Verification items for the finished model (mm, model axes). Face numbers are marked on the shaded views. A direction names the side the tool comes from. Round coordinates to 2 decimals unless told otherwise and drop trailing zeros. Write each loop counter-clockwise with the first axis right and the second up, starting at its lowest first coordinate (ties: lowest second). Pieces come first, ordered by that corner, then holes. Notation, with made-up numbers: M 41.5,4.5 L 83.5,4.5 A20 cw 83.5,39.5 Z; hole C -8,-14 d3. An arc over 180 degrees is marked long. One line per item, written item: value. Start each with the question number.
from build123d import *

# Parameters (mm, degrees)
F0_W     = 19.2
F0_H     = 100
F1_DEPTH = 19.2
F2_W     = 15.4
F2_H     = 15.4
F3_DEPTH = 18
F4_SIZE  = 0.5


# Not quite as in the source:
# - a pattern or mirror of a feature is missing from the dataset's text; its kind, count and spacing are read off the source's solid


with BuildPart() as f1:
    # F0 (on Top) → F1 (new body)
    with BuildSketch(Plane.XY):
        Rectangle(F0_W, F0_H)
    extrude(amount=F1_DEPTH)

    # F2 (on face) → F3 (cut)
    with BuildSketch(Plane.YZ.offset(9.6)):
        with Locations((-40.4, 9.6)):
            Rectangle(F2_W, F2_H)
    f3 = extrude(amount=-F3_DEPTH, mode=Mode.SUBTRACT)

    # F3_copies: F3 across plane
    add(f3.mirror(Plane.ZX), mode=Mode.SUBTRACT)

    # F4
    f4_edges = [f1.edges().sort_by_distance(p)[0] for p in [
        (-9.6, 50, 9.6),
        (-9.6, -50, 9.6),
        (-9.6, 0, 0),
        (-9.6, 0, 19.2),
        (0, -50, 19.2),
        (9.6, 0, 19.2),
        (0, 50, 19.2),
        (9.6, -50, 9.6),
        (0, -50, 0),
        (9.6, 0, 0),
        (0, 50, 0),
        (9.6, 50, 9.6),
    ]]
    chamfer(f4_edges, length=F4_SIZE)


solid = f1.part
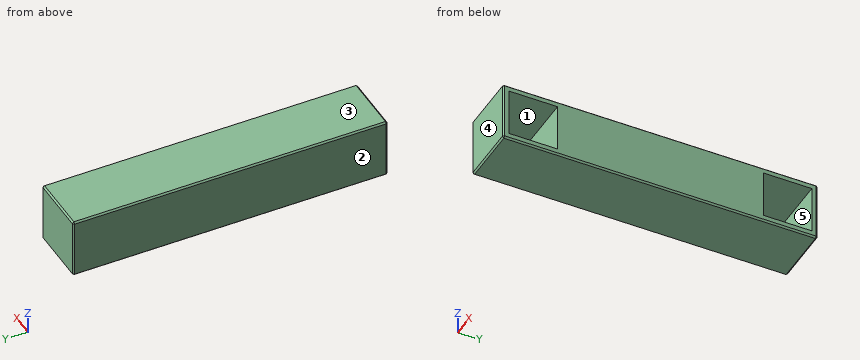
1) Cross-section at C-C (z = 13). Record the boundary of the cut face in (x, y).
2) Thickness scan on line 1 (Y direction, x = 7, z = 6); line 2 (Z direction, x = 3.75, y = 40). Record the ranges inside material, lowest first.
3) Cross-section at A-A (x = -7). Record the boundary of the cut face in (y, z).
4) Cross-section at B-B (y = 34). Record the boundary of the cut face in (x, z), then the cut area to 3 significant figures.
5) Access from +Z, -Z, +X, -X, +Y, -Y to the whole of each face (thin tool, end or side, straight path). Record for the marked faces 1 and 2.
6) Mould release check, pull along Z, two halves, no side actions. Record for the marked faces 3, 4 and 5: pulls with the +Z half, pulls with the -Z half, needs draft (parallel to the pull), parting line crosses it, or undercut.
Results below:
1. outline: M -9.6,-49.5 L -9.1,-50 L 9.1,-50 L 9.6,-49.5 L 9.6,-48.1 L -8.4,-48.1 L -8.4,-32.7 L 9.6,-32.7 L 9.6,32.7 L -8.4,32.7 L -8.4,48.1 L 9.6,48.1 L 9.6,49.5 L 9.1,50 L -9.1,50 L -9.6,49.5 Z
2. line 1: y = -50 to -48.1, -32.7 to 32.7, 48.1 to 50
2. line 2: z = 0 to 1.9, 17.3 to 19.2
3. outline: M -50,0.5 L -49.5,0 L 49.5,0 L 50,0.5 L 50,18.7 L 49.5,19.2 L -49.5,19.2 L -50,18.7 Z; hole M -48.1,1.9 L -32.7,1.9 L -32.7,17.3 L -48.1,17.3 Z; hole M 32.7,1.9 L 48.1,1.9 L 48.1,17.3 L 32.7,17.3 Z
4. outline: M -9.6,0.5 L -9.1,0 L 9.1,0 L 9.6,0.5 L 9.6,1.9 L -8.4,1.9 L -8.4,17.3 L 9.6,17.3 L 9.6,18.7 L 9.1,19.2 L -9.1,19.2 L -9.6,18.7 Z
4. area: 90.9 mm²
5. face 1: +X
5. face 2: +Z, -Z, -X, +Y, -Y
6. face 3: pulls with the +Z half
6. face 4: needs draft
6. face 5: undercut
